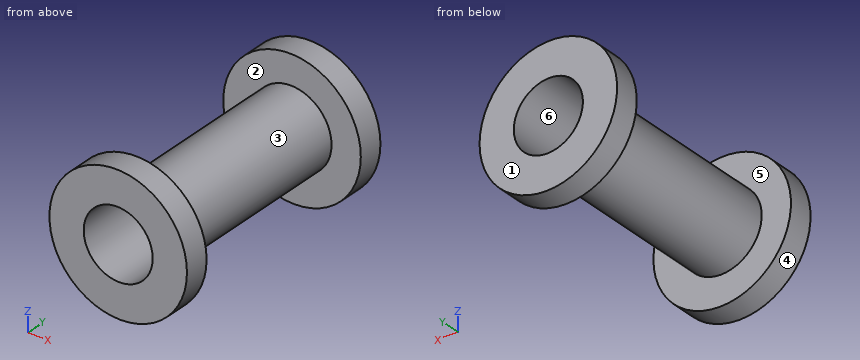
from build123d import *

# Parameters (mm, degrees)
SKETCH1_R      = 20.066
SKETCH1_R_2    = 17.526
EXTRUDE1_DEPTH = 125.222
SKETCH2_R      = 34.925
SKETCH2_R_2    = 17.526
EXTRUDE2_DEPTH = 12.7
SKETCH3_R      = 34.925
SKETCH3_R_2    = 17.526
EXTRUDE3_DEPTH = 12.7


with BuildPart() as part:
    # Sketch1 → Extrude1 (new body)
    with BuildSketch(Plane(origin=(0, 0, 0), x_dir=(1, 0, 0), z_dir=(0, 1, 0))):
        Circle(SKETCH1_R)
        Circle(SKETCH1_R_2, mode=Mode.SUBTRACT)
    extrude(amount=EXTRUDE1_DEPTH)

    # Sketch2 → Extrude2 (add)
    with BuildSketch(Plane(origin=(0, 125.222, 0), x_dir=(1, 0, 0), z_dir=(0, 1, 0))):
        Circle(SKETCH2_R)
        Circle(SKETCH2_R_2, mode=Mode.SUBTRACT)
    extrude(amount=-EXTRUDE2_DEPTH)

    # Sketch3 → Extrude3 (add)
    with BuildSketch(Plane.XZ):
        Circle(SKETCH3_R)
        Circle(SKETCH3_R_2, mode=Mode.SUBTRACT)
    extrude(amount=-EXTRUDE3_DEPTH)


solid = part.part
Could you check a few things on this model? Use its own coordinates, in mm. Face numbers are marked on the shaded views. A direction names the side the tool comes from. Round coordinates to 2 decimals unless told otherwise and drop trailing zeros. Write each loop counter-clockwise with the first axis right and the second up, starting at its lowest first coordinate (ties: lowest second). Pieces come first, ordered by that corner, then holes. Notation, with made-up numbers: (47.5, 46) -> (60.5, 46) arc R13 ccw to (60.5, 66) -> close; hole circle Ø6 at (45.5, 44). An arc over 180 degrees is marked (long way). Use a Markdown table: item, result.
1. Please list where these lines run through material, in increasing order: probe 1 along Y at (x, z) = (30.5, 2.5); probe 2 along Z at (x, y) = (0, 27); probe 3 along X at (y, z) = (13, -15).
Answer key:
| item | result |
|---|---|
| probe 1 | y = 0 to 12.7, 112.52 to 125.22 |
| probe 2 | z = -20.07 to -17.53, 17.53 to 20.07 |
| probe 3 | x = -13.33 to -9.06, 9.06 to 13.33 |
2. If we section it at A-A (z = 0): List the corners of the cut face in (x, y) for me (3 decimals).
Answer key:
| item | result |
|---|---|
| outline | (-34.925, 0) -> (-17.526, 0) -> (-17.526, 125.222) -> (-34.925, 125.222) -> (-34.925, 112.522) -> (-20.066, 112.522) -> (-20.066, 12.7) -> (-34.925, 12.7) -> close; (17.526, 0) -> (34.925, 0) -> (34.925, 12.7) -> (20.066, 12.7) -> (20.066, 112.522) -> (34.925, 112.522) -> (34.925, 125.222) -> (17.526, 125.222) -> close |
3. If we section it at B-B (x = 0): List the corners of the cut face in (y, z) for me (3 decimals).
Answer key:
| item | result |
|---|---|
| outline | (0, -34.925) -> (12.7, -34.925) -> (12.7, -20.066) -> (112.522, -20.066) -> (112.522, -34.925) -> (125.222, -34.925) -> (125.222, -17.526) -> (0, -17.526) -> close; (0, 17.526) -> (125.222, 17.526) -> (125.222, 34.925) -> (112.522, 34.925) -> (112.522, 20.066) -> (12.7, 20.066) -> (12.7, 34.925) -> (0, 34.925) -> close |
4. We'd pull the mould along Y, two halves only. Please class the marked faces 1, 2, 3 and 4: +Y half, -Y half, draft (parallel to the pull), parting line (faces both ways), or undercut.
Answer key:
| item | result |
|---|---|
| face 1 | +Y half |
| face 2 | undercut |
| face 3 | undercut |
| face 4 | draft |
5. If we section it at D-D (x = -31): List the corners of the cut face in (y, z) for me.
Answer key:
| item | result |
|---|---|
| outline | (0, -16.09) -> (12.7, -16.09) -> (12.7, 16.09) -> (0, 16.09) -> close; (112.52, -16.09) -> (125.22, -16.09) -> (125.22, 16.09) -> (112.52, 16.09) -> close |
6. For pin 1 Ø2 at (y, z) = (92, 2) entering from -X; pin 2 Ø2 at (y, z) = (21.5, 17) entering from -X; pin 3 Ø10 at (y, z) = (26, -9) entering from +X, each with a flat end and sliding along its axis, tell me the tip position at first contact or that it passes through.
Answer key:
| item | result |
|---|---|
| pin 1 | stops at x = -20.04 |
| pin 2 | stops at x = -12.11 |
| pin 3 | stops at x = 19.66 |
7. Which directions (+Z, -Z, +X, -X, +Y, -Y) give clear straight access to the entire face, cutting with the end or side of a thin tool? Please do the marked faces 5 and 6.
Answer key:
| item | result |
|---|---|
| face 5 | none |
| face 6 | +Y, -Y |
8. If we section it at C-C (y = 64): List the corners of the cut face in (x, z) for me, then the cut area to 3 significant figures.
Answer key:
| item | result |
|---|---|
| outline | circle Ø40.13 at (0, 0); hole circle Ø35.05 at (0, 0) |
| area | 300 mm^2 |
